Check sheet for the modelled part. Datum: model origin and axes. Units: mm. Face numbers are marked on the shaded views. A direction names the side the tool comes from. Round coordinates to 2 decimals unless told otherwise and drop trailing zeros. Write each loop counter-clockwise with the first axis right and the second up, starting at its lowest first coordinate (ties: lowest second). Pieces come first, ordered by that corner, then holes.
Item 1: Section check D-D, the plane x = -10. Record the cut outline in (y, z) (1 decimal), plus the area to 3 significant figures.
Item 2: Set-up check for the marked faces 1 and 2: record each of +Z, -Z, +X, -X, +Y, -Y from which the full face is reachable in a straight line by a thin tool's end or side.
Item 3: Material ranges on line 1 along Y through (x, z) = (0, 1); line 2 along X through (y, z) = (-21, 1.4); line 3 along X through (y, z) = (-26, 0.85), recorded low to high.
Item 4: Depth check by flat-ended pin: pin 1 (1.5 mm diameter, centred on x = 15, z = 1.5, fed in from -Y); pin 2 (0.5 mm diameter, centred on y = 25, z = 1, fed in from -X); pin 3 (4 mm diameter, centred on x = -4, y = -24.5, fed in from +Z). Enter the tip coordinate at first touch or a pass-through.
Item 5: Section check B-B, the plane z = 2.2. Record the cut outline in (x, y), plus the area to 3 significant figures.
Item 6: Section check A-A, the plane x = 0. Record the cut outline in (y, z), plus the area to 3 significant figures.
Item 7: Section check C-C, the plane y = 10.5. Record the cut outline in (x, z) (1 decimal), plus the area to 3 significant figures.
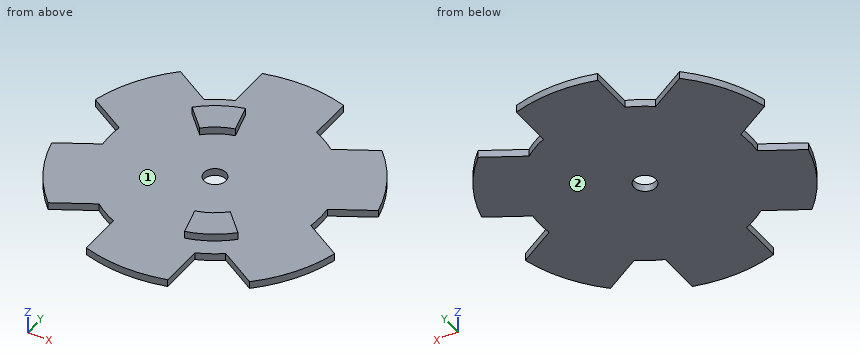
from build123d import *

# Parameters (mm, degrees)
EXTRUDE1_DEPTH      = 1.5875
SKETCH2_R           = 2.38125
CUT_EXTRUDE1_DEPTH  = 2.5875
BOSS_EXTRUDE1_DEPTH = 1.5875


with BuildPart() as part:
    # Sketch1 → Extrude1 (new body)
    with BuildSketch(Plane.XY):
        with BuildLine():
            Line((22.679380466, 2.841623674), (30.838674439, 7.552394246))
            ThreePointArc((30.838674439, 7.552394246), (27.49630657, 15.875), (21.959902496, 22.93087836))
            Line((21.959902496, 22.93087836), (13.800608523, 18.220107788))
            ThreePointArc((13.800608523, 18.220107788), (11.428354249, 19.794490207), (8.878771943, 21.061731462))
            Line((8.878771943, 21.061731462), (8.878771943, 30.483272606))
            ThreePointArc((8.878771943, 30.483272606), (0, 31.75), (-8.878771943, 30.483272606))
            Line((-8.878771943, 30.483272606), (-8.878771943, 21.061731462))
            ThreePointArc((-8.878771943, 21.061731462), (-11.42835425, 19.794490207), (-13.800608523, 18.220107788))
            Line((-13.800608523, 18.220107788), (-21.959902496, 22.93087836))
            ThreePointArc((-21.959902496, 22.93087836), (-27.49630657, 15.875), (-30.838674439, 7.552394246))
            Line((-30.838674439, 7.552394246), (-22.679380466, 2.841623674))
            ThreePointArc((-22.679380466, 2.841623674), (-22.856708499, 0), (-22.679380466, -2.841623674))
            Line((-22.679380466, -2.841623674), (-30.838674439, -7.552394246))
            ThreePointArc((-30.838674439, -7.552394246), (-27.49630657, -15.875), (-21.959902496, -22.93087836))
            Line((-21.959902496, -22.93087836), (-13.800608523, -18.220107788))
            ThreePointArc((-13.800608523, -18.220107788), (-11.428354249, -19.794490207), (-8.878771943, -21.061731462))
            Line((-8.878771943, -21.061731462), (-8.878771943, -30.483272606))
            ThreePointArc((-8.878771943, -30.483272606), (0, -31.75), (8.878771943, -30.483272606))
            Line((8.878771943, -30.483272606), (8.878771943, -21.061731462))
            ThreePointArc((8.878771943, -21.061731462), (11.42835425, -19.794490207), (13.800608523, -18.220107788))
            Line((13.800608523, -18.220107788), (21.959902496, -22.93087836))
            ThreePointArc((21.959902496, -22.93087836), (27.49630657, -15.875), (30.838674439, -7.552394246))
            Line((30.838674439, -7.552394246), (22.679380466, -2.841623674))
            ThreePointArc((22.679380466, -2.841623674), (22.856708499, 0), (22.679380466, 2.841623674))
        make_face()
    extrude(amount=EXTRUDE1_DEPTH)

    # Sketch2 → Cut-Extrude1 (cut, through all)
    with BuildSketch(Plane.XY.offset(1.5875)):
        Circle(SKETCH2_R)
    extrude(amount=-CUT_EXTRUDE1_DEPTH, mode=Mode.SUBTRACT)

    # Sketch3 → Boss-Extrude1 (add)
    with BuildSketch(Plane.XY.offset(1.5875)):
        with BuildLine():
            Line((-13.470384182, 13.470384182), (-8.980256121, 8.980256121))
            ThreePointArc((-8.980256121, 8.980256121), (-6.35, 10.998522628), (-3.287001873, 12.267257994))
            Line((-3.287001873, 12.267257994), (-4.930502809, 18.400886991))
            ThreePointArc((-4.930502809, 18.400886991), (-9.525, 16.497783942), (-13.470384182, 13.470384182))
        make_face()
        with BuildLine():
            Line((13.470384182, -13.470384182), (8.980256121, -8.980256121))
            ThreePointArc((8.980256121, -8.980256121), (6.35, -10.998522628), (3.287001873, -12.267257994))
            Line((3.287001873, -12.267257994), (4.930502809, -18.400886991))
            ThreePointArc((4.930502809, -18.400886991), (9.525, -16.497783942), (13.470384182, -13.470384182))
        make_face()
    extrude(amount=BOSS_EXTRUDE1_DEPTH)


solid = part.part
Values found:
1. outline: (-20.6, 0) - (20.6, 0) - (20.6, 1.6) - (16.2, 1.6) - (16.2, 3.2) - (10, 3.2) - (10, 1.6) - (-20.6, 1.6) - close
1. area: 75.1 mm2
2. face 1: +Z
2. face 2: -Z, +X, -X, +Y, -Y
3. line 1: y = -31.75 to -2.38, 2.38 to 31.75
3. line 2: x = -23.81 to -18.62, -9.02 to 9.02, 18.62 to 23.81
3. line 3: x = -8.88 to 8.88
4. pin 1: stops at y = -19.35
4. pin 2: stops at x = -8.88
4. pin 3: stops at z = 1.59
5. outline: (-13.47, 13.47) - (-8.98, 8.98) arc R12.7 cw to (-3.29, 12.27) - (-4.93, 18.4) arc R19.05 ccw to start; (3.29, -12.27) - (4.93, -18.4) arc R19.05 ccw to (13.47, -13.47) - (8.98, -8.98) arc R12.7 cw to start
5. area: 106 mm2
6. outline: (-31.75, 0) - (-2.38, 0) - (-2.38, 1.59) - (-31.75, 1.59) - close; (2.38, 0) - (31.75, 0) - (31.75, 1.59) - (2.38, 1.59) - close
6. area: 93.2 mm2
7. outline: (-30, 0) - (30, 0) - (30, 1.6) - (-7.1, 1.6) - (-7.1, 3.2) - (-10.5, 3.2) - (-10.5, 1.6) - (-30, 1.6) - close
7. area: 100 mm2
